from build123d import *

# Parameters (mm, degrees)
MODEL_R                 = 5.602685567
MODEL_R_2               = 2
MODEL_W                 = 10
MODEL_H                 = 3
SALIENTE_EXTRUIR1_DEPTH = 3


with BuildPart() as part:
    # Model → Saliente-Extruir1 (new body)
    with BuildSketch(Plane.XY):
        with BuildLine():
            Line((-237.074609356, -49.671573713), (-258.074609356, -49.671573713))
            Line((-258.074609356, -49.671573713), (-258.074609356, 13.328426287))
            ThreePointArc((-258.074609356, 13.328426287), (-256.610143262, 16.863960193), (-253.074609356, 18.328426287))
            Line((-253.074609356, 18.328426287), (-242.074609356, 18.328426287))
            Line((-242.074609356, 18.328426287), (-212.074609356, 48.328426287))
            Line((-212.074609356, 48.328426287), (-162.074609356, 48.328426287))
            Line((-162.074609356, 48.328426287), (-132.074609356, 18.328426287))
            Line((-132.074609356, 18.328426287), (-121.074609356, 18.328426287))
            ThreePointArc((-121.074609356, 18.328426287), (-117.53907545, 16.863960193), (-116.074609356, 13.328426287))
            Line((-116.074609356, 13.328426287), (-116.074609356, -49.671573713))
            Line((-116.074609356, -49.671573713), (-137.074609356, -49.671573713))
            Line((-137.074609356, -49.671573713), (-137.074609356, -38.671573713))
            Line((-137.074609356, -38.671573713), (-132.574609356, -38.671573713))
            Line((-132.574609356, -38.671573713), (-132.574609356, -30.671573713))
            Line((-132.574609356, -30.671573713), (-137.074609356, -30.671573713))
            Line((-137.074609356, -30.671573713), (-137.074609356, -24.671573713))
            Line((-137.074609356, -24.671573713), (-148.074609356, -24.671573713))
            Line((-148.074609356, -24.671573713), (-148.074609356, -30.671573713))
            Line((-148.074609356, -30.671573713), (-152.574609356, -30.671573713))
            Line((-152.574609356, -30.671573713), (-152.574609356, -38.671573713))
            Line((-152.574609356, -38.671573713), (-148.074609356, -38.671573713))
            Line((-148.074609356, -38.671573713), (-148.074609356, -49.671573713))
            Line((-148.074609356, -49.671573713), (-226.074609356, -49.671573713))
            Line((-226.074609356, -49.671573713), (-226.074609356, -38.671573713))
            Line((-226.074609356, -38.671573713), (-221.574609356, -38.671573713))
            Line((-221.574609356, -38.671573713), (-221.574609356, -30.671573713))
            Line((-221.574609356, -30.671573713), (-226.074609356, -30.671573713))
            Line((-226.074609356, -30.671573713), (-226.074609356, -24.671573713))
            Line((-226.074609356, -24.671573713), (-237.074609356, -24.671573713))
            Line((-237.074609356, -24.671573713), (-237.074609356, -30.671573713))
            Line((-237.074609356, -30.671573713), (-241.574609356, -30.671573713))
            Line((-241.574609356, -30.671573713), (-241.574609356, -38.671573713))
            Line((-241.574609356, -38.671573713), (-237.074609356, -38.671573713))
            Line((-237.074609356, -38.671573713), (-237.074609356, -49.671573713))
        make_face()
        with Locations((-231.074609356, 2.328426287)):
            Circle(MODEL_R, mode=Mode.SUBTRACT)
        with Locations((-143.074609356, 2.328426287)):
            Circle(MODEL_R, mode=Mode.SUBTRACT)
        with Locations((-168.074609356, 41.328426287)):
            Circle(MODEL_R_2, mode=Mode.SUBTRACT)
        with Locations((-206.074609356, 41.328426287)):
            Circle(MODEL_R_2, mode=Mode.SUBTRACT)
        Polygon((-157.905285481, 31.673821038), (-150.834217669, 24.602753226), (-148.712897325, 26.724073569), (-155.783965137, 33.795141381), align=None, mode=Mode.SUBTRACT)
        Polygon((-250.185058728, -2.267304459), (-243.113990916, 4.803763352), (-245.23531126, 6.925083696), (-252.306379072, -0.145984116), align=None, mode=Mode.SUBTRACT)
        with Locations((-206.074609356, 32.328426287)):
            Rectangle(MODEL_W, MODEL_H, mode=Mode.SUBTRACT)
        Polygon((-123.964159984, -2.267304459), (-131.035227796, 4.803763352), (-128.913907452, 6.925083696), (-121.84283964, -0.145984116), align=None, mode=Mode.SUBTRACT)
        Polygon((-216.243933231, 31.673821038), (-223.315001043, 24.602753226), (-225.436321387, 26.724073569), (-218.365253575, 33.795141381), align=None, mode=Mode.SUBTRACT)
        with Locations((-168.074609356, 32.328426287)):
            Rectangle(MODEL_W, MODEL_H, mode=Mode.SUBTRACT)
    extrude(amount=SALIENTE_EXTRUIR1_DEPTH)


solid = part.part
Source: CAD feature listing. Evaluate the final solid. Frame: model axes, mm. A direction names the side the tool comes from. Give positions to 0.01 mm unless a question says otherwise; leave off trailing zeros. Order: outer loops, then holes, each group sorted by start corner. A loop starts at its lowest first (then second) coordinate and runs counter-clockwise, first axis right, second up. Notation, with made-up numbers: (77.25, -7.5) -> (128.25, -7.5) arc R15 cw to (128.25, 16.5) -> close; hole circle Ø6 at (-25.75, 17.5). An arc over 180 degrees is marked (long way). Write item = value, one per line.
Q1. Pin query (flat end, axial travel): pin 1 (1.5 mm diameter, centred on y = 32, z = 1.5, fed in from +X); pin 2 (1.5 mm diameter, centred on y = 32.5, z = 2, fed in from -X); pin 3 (6.5 mm diameter, centred on x = -143.07, y = 2.33, fed in from -Z); pin 4 (0.9 mm diameter, centred on y = 32, z = 1.5, fed in from -X). Return the tip coordinate at first contact, or that it passes through.
Data:
pin_1 = -145
pin_2 = -228.65
pin_3 = through
pin_4 = -228.85
Q2. Pull-direction query (Y, two-part tool) for faces 1 (the face through (-239, -30.672, 1)), 2 (the face through (-258.075, -19, 1)), 3 (the face through (-227.285, 33.118, 1.479)); classes: released by +Y, released by -Y, zero draft, split by the parting line, or undercut.
Data:
face_1 = undercut
face_2 = zero draft
face_3 = released by +Y
Q3. Set-up query: faces 4 (the face through (-248.72, 3.44, 1.48)), 5 (the face through (-127, 18.328, 1)), 6 (the face through (-226.075, -44, 1)). Return all of +Z, -Z, +X, -X, +Y, -Y with unobstructed straight access to the full face (end or side cutting, diameter ignored); none if empty.
Data:
face_4 = +Z, -Z
face_5 = +Z, -Z, +X, +Y
face_6 = +Z, -Z, -Y
Q4. Material intervals for line 1 (X direction, y = -34.5, z = 2.25); line 2 (X direction, y = -40.5, z = 0.4); line 3 (X direction, y = -2, z = 1.9), sorted ascending. Write a range as from..to.
Data:
line_1 = -258.07..-241.57, -221.57..-152.57, -132.57..-116.07
line_2 = -258.07..-237.07, -226.07..-148.07, -137.07..-116.07
line_3 = -258.07..-250.45, -249.92..-234.63, -227.52..-146.63, -139.52..-124.23, -123.7..-116.07
Q5. Cut plane B-B, the plane z = 0.6. State how many separate pieces and enclosed holes the cut face has, and give its area (3 significant figures).
Data:
separate_pieces = 1
enclosed_holes = 10
area = 10,900 mm^2
Q6. Cut plane A-A, the plane x = -164.5. Output: boundary loops of the cut face in (y, z).
Data:
outline = (-49.67, 0) -> (30.83, 0) -> (30.83, 3) -> (-49.67, 3) -> close; (33.83, 0) -> (48.33, 0) -> (48.33, 3) -> (33.83, 3) -> close
